Input: dimensioned drawing with shaded views. Units: mm. Origin: part minimum x, y, z. A direction names the side the tool comes from. Give positions to 0.01 mm unless a question says otherwise; leave off trailing zeros. Write each loop counter-clockwise with the first axis right and the second up, starting at its lowest first coordinate (ties: lowest second). Pieces come first, ordered by that corner, then holes. Notation, with made-up numbers: M 38.25,57.25 L 89.25,57.25 A22 ccw 89.25,94.25 Z; hole C -33,-38 d5. An arc over 180 degrees is marked long. Use CSV: the item, a comma, the result in double quotes. Start each with the question number.
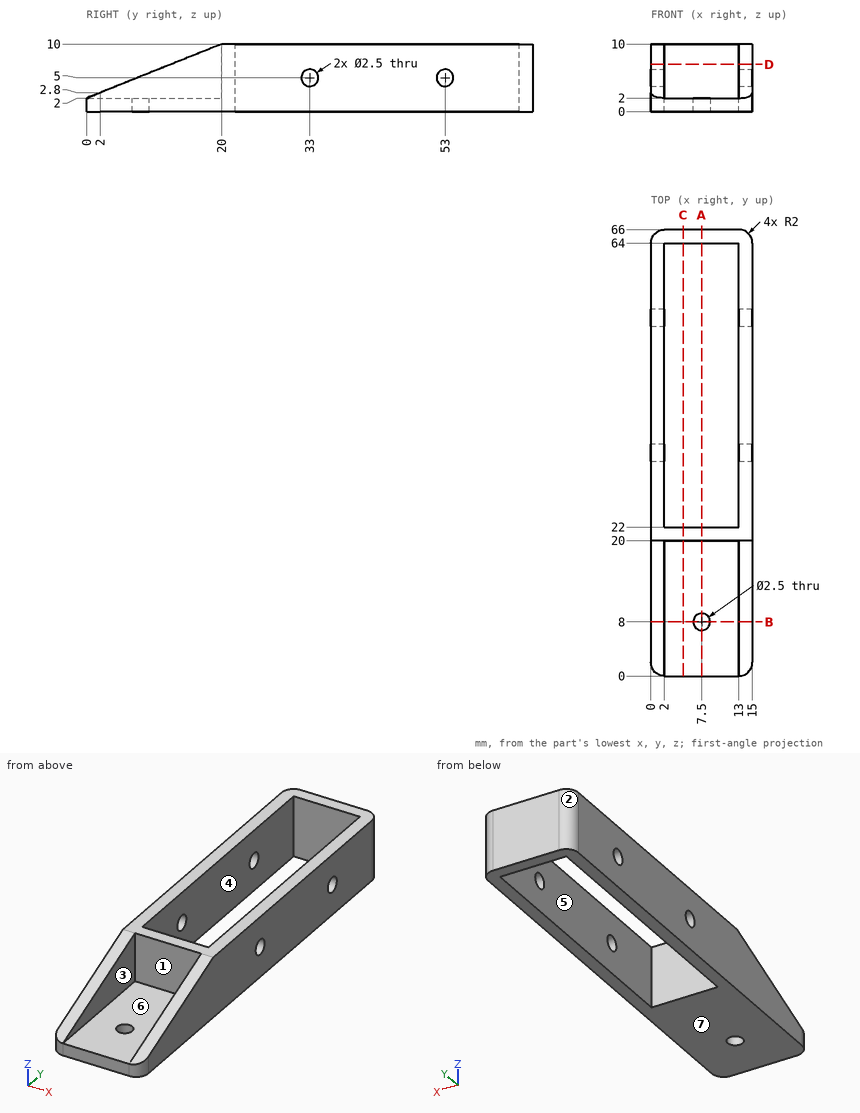
Item 1: Contact query for a flat-ended pin moving along its axis: pin 1 Ø9 at (x, y) = (8, 6) entering from +Z. Output: stop coordinate, or through.
Item 2: Section D-D (z = 7). Return the cut outline in (x, y).
Item 3: Section A-A (x = 7.5). Return the cut outline in (y, z).
Item 4: Pull-direction query (Y, two-part tool) for the marked faces 1, 2, 3 and 4; classes: released by +Y, released by -Y, zero draft, split by the parting line, or undercut.
Item 5: Set-up query: the marked faces 5, 6 and 7. Return all of +Z, -Z, +X, -X, +Y, -Y with unobstructed straight access to the full face (end or side cutting, diameter ignored); none if empty.
Item 6: Section C-C (x = 4.75). Return the cut outline in (y, z), plus the area to 3 significant figures.
Item 7: Material intervals for probe 1 along X at (y, z) = (52, 7.5); probe 2 along Y at (x, z) = (8.5, 4.5); probe 3 along Y at (x, z) = (7.5, 1.15), sorted ascending.
Item 8: Section B-B (y = 8). Return the cut outline in (x, z), plus the area to 3 significant figures.
Output values:
1,pin 1,"stops at z = 2"
2,outline,"M 0,12.5 L 2,12.5 L 2,20 L 13,20 L 13,12.5 L 15,12.5 L 15,64 A2 ccw 13,66 L 2,66 A2 ccw 0,64 Z; hole M 2,22 L 13,22 L 13,64 L 2,64 Z"
3,outline,"M 0,0 L 6.75,0 L 6.75,2 L 0,2 Z; M 9.25,0 L 22,0 L 22,10 L 20,10 L 20,2 L 9.25,2 Z; M 64,0 L 66,0 L 66,10 L 64,10 Z"
4,face 1,"released by -Y"
4,face 2,"released by +Y"
4,face 3,"zero draft"
4,face 4,"undercut"
5,face 5,"+Z, -Z"
5,face 6,"+Z, -Y"
5,face 7,"-Z, +X, -X, +Y, -Y"
6,outline,"M 0,0 L 22,0 L 22,10 L 20,10 L 20,2 L 0,2 Z; M 64,0 L 66,0 L 66,10 L 64,10 Z"
6,area,"80.0 mm2"
7,probe 1,"x = 0 to 2, 13 to 15"
7,probe 2,"y = 20 to 22, 64 to 66"
7,probe 3,"y = 0 to 6.75, 9.25 to 22, 64 to 66"
8,outline,"M 0,0 L 6.25,0 L 6.25,2 L 2,2 L 2,5.2 L 0,5.2 Z; M 8.75,0 L 15,0 L 15,5.2 L 13,5.2 L 13,2 L 8.75,2 Z"
8,area,"37.8 mm2"
